Can you work these out from the model? Positions are in its coordinate system, mm. A direction names the side the tool comes from. Coordinates: 2 decimals unless noted, no trailing zeros. Write each loop counter-clockwise with the first axis right and the second up, starting at its lowest first coordinate (ties: lowest second). Pieces come first, ordered by that corner, then holes. Notation, with made-up numbers: (-12, 77) - (36, 77) arc R10 ccw to (36, 94) - close; hole circle Ø5 at (80, -11). An arc over 180 degrees is marked (long way). Use one line per item in the form item = value. Start each with the question number.
(1) On a 3-axis mill with a long thin cutter (end or side, diameter ignored), from which of +Z, -Z, +X, -X, +Y, -Y can I reach the whole of each face in a straight line? I mean faces 4 (the face through (40, 0, -4)), 5 (the face through (-31.773, -1.734, -2.076)), 6 (the face through (61.238, 19.194, -29.126)). Say none if no direction works.
(2) Thinking about a two-plate mould opening in Z: for faces 1 (the face through (-1, -30, -16)), 2 (the face through (32.064, -1.734, -2.076)), 3 (the face through (-55, 0, -19.266)), which applies, pulls with the +Z half, pulls with the -Z half, needs draft (parallel to the pull), parting line crosses it, or undercut?
(3) If we section it at B-B on y = -16.5: Please give me the cut outline in (x, z).
(4) If we section it at C-C on y = 22.5: Please give me the cut outline in (x, z), then the cut area to 3 significant figures.
(5) If we section it at A-A on y = 2.5: Please give me the cut outline in (x, z).
(6) For pin 1 Ø8 at (y, z) = (10, 5) entering from -X; pin 2 Ø6 at (y, z) = (-16.5, 12) entering from +X; pin 3 Ø12 at (x, y) = (4.5, -2) entering from +Z, each with a flat end and sliding along its axis, tell me the tip position at first contact or that it passes through.
(7) If we section it at D-D on x = 0: Please give me the cut outline in (y, z).
(8) If I drill on probe 1 along X at (y, z) = (2, -23); probe 2 along X at (y, z) = (18, -34.5); probe 3 along X at (y, z) = (-6.5, -19), over which ranges is the centre line in solid material (lowest first)? Write a range as from..to.
```python
from build123d import *

# Parameters (mm, degrees)
F1_DEPTH = 30
F2_R     = 8
F3_DEPTH = 120.001
F5_DEPTH = 20.001
F7_DEPTH = 20.001


with BuildPart() as f1:
    # F0 (on Front) → F1 (new body, symmetric)
    with BuildSketch(Plane.XZ):
        with BuildLine():
            Line((-80, -39.266379), (80, -39.266379))
            Line((80, -39.266379), (80, -19.266379))
            Line((80, -19.266379), (40, -19.266379))
            Line((40, -19.266379), (40, 20.733621))
            Line((40, 20.733621), (30, 20.733621))
            ThreePointArc((30, 20.733621), (0, -9.266379), (-30, 20.733621))
            Line((-30, 20.733621), (-40, 20.733621))
            Line((-40, 20.733621), (-40, -19.266379))
            Line((-40, -19.266379), (-80, -19.266379))
            Line((-80, -19.266379), (-80, -39.266379))
        make_face()
    extrude(amount=F1_DEPTH, both=True)

    # F2 (on face) → F3 (cut, through all)
    with BuildSketch(Plane.YZ.offset(40)):
        with Locations((0, 5.733621)):
            Circle(F2_R)
    extrude(amount=-F3_DEPTH, mode=Mode.SUBTRACT)

    # F4 (on face) → F5 (cut, through all)
    with BuildSketch(Plane.XY.offset(-19.266379)):
        with BuildLine():
            ThreePointArc((-58.471588, 15), (-60.228947, 19.242641), (-64.471588, 21))
            Line((-64.471588, 21), (-65, 21))
            ThreePointArc((-65, 21), (-69.242641, 19.242641), (-71, 15))
            Line((-71, 15), (-71, -15))
            ThreePointArc((-71, -15), (-69.242641, -19.242641), (-65, -21))
            Line((-65, -21), (-64.471588, -21))
            ThreePointArc((-64.471588, -21), (-60.228947, -19.242641), (-58.471588, -15))
            Line((-58.471588, -15), (-58.471588, 15))
        make_face()
    extrude(amount=-F5_DEPTH, mode=Mode.SUBTRACT)

    # F6 (on face) → F7 (cut, through all)
    with BuildSketch(Plane.XY.offset(-19.266379)):
        with BuildLine():
            ThreePointArc((71, 15), (69.335045, 19.148178), (65.264206, 20.99418))
            ThreePointArc((65.264206, 20.99418), (61.193367, 19.148178), (59.528412, 15))
            Line((59.528412, 15), (59.528412, -15))
            ThreePointArc((59.528412, -15), (61.193367, -19.148178), (65.264206, -20.99418))
            ThreePointArc((65.264206, -20.99418), (69.335045, -19.148178), (71, -15))
            Line((71, -15), (71, 15))
        make_face()
    extrude(amount=-F7_DEPTH, mode=Mode.SUBTRACT)


solid = f1.part
```
Reported:
q1.face_4 = +Z, +X, +Y, -Y
q1.face_5 = +X, -X
q1.face_6 = +Z, -Z
q2.face_1 = needs draft
q2.face_2 = undercut
q2.face_3 = pulls with the +Z half
q3.outline = (-80, -39.27) - (-70.81, -39.27) - (-70.81, -19.27) - (-80, -19.27) - close; (-58.66, -39.27) - (59.72, -39.27) - (59.72, -19.27) - (40, -19.27) - (40, 20.73) - (30, 20.73) arc R30 cw to (-30, 20.73) - (-40, 20.73) - (-40, -19.27) - (-58.66, -19.27) - close; (70.81, -39.27) - (80, -39.27) - (80, -19.27) - (70.81, -19.27) - close
q4.outline = (-80, -39.27) - (80, -39.27) - (80, -19.27) - (40, -19.27) - (40, 20.73) - (30, 20.73) arc R30 cw to (-30, 20.73) - (-40, 20.73) - (-40, -19.27) - (-80, -19.27) - close
q4.area = 4,990 mm2
q5.outline = (-80, -39.27) - (-71, -39.27) - (-71, -19.27) - (-80, -19.27) - close; (-58.47, -39.27) - (59.53, -39.27) - (59.53, -19.27) - (40, -19.27) - (40, -1.87) - (19.73, -1.87) arc R30 cw to (-19.73, -1.87) - (-40, -1.87) - (-40, -19.27) - (-58.47, -19.27) - close; (-40, 13.33) - (-29.07, 13.33) arc R30 cw to (-30, 20.73) - (-40, 20.73) - close; (29.07, 13.33) - (40, 13.33) - (40, 20.73) - (30, 20.73) arc R30 cw to start; (71, -39.27) - (80, -39.27) - (80, -19.27) - (71, -19.27) - close
q6.pin_1 = -40
q6.pin_2 = 40
q6.pin_3 = -7.37
q7.outline = (-30, -39.27) - (30, -39.27) - (30, -9.27) - (-30, -9.27) - close
q8.probe_1 = -80..-71, -58.47..59.53, 71..80
q8.probe_2 = -80..-70.2, -59.28..60.33, 70.2..80
q8.probe_3 = -40..40
